from build123d import *

# Parameters (mm, degrees)
SKETCH2_R      = 3.405
EXTRUDE1_DEPTH = 550


with BuildPart() as part:
    # Sketch2 → Extrude1 (new, symmetric)
    with BuildSketch(Plane.XY):
        with BuildLine():
            Line((-16.82, 20), (-5.635, 20))
            ThreePointArc((-5.635, 20), (-4.524842354, 19.540157646), (-4.065, 18.43))
            Line((-4.065, 18.43), (-4.065, 17.51))
            ThreePointArc((-4.065, 17.51), (-4.524842354, 16.399842354), (-5.635, 15.94))
            Line((-5.635, 15.94), (-6.855, 15.94))
            Line((-6.855, 15.94), (-6.855, 16.77))
            Line((-6.855, 16.77), (-9.015, 16.77))
            ThreePointArc((-9.015, 16.77), (-9.913025612, 16.398025612), (-10.285, 15.5))
            Line((-10.285, 15.5), (-10.285, 12.987102448))
            ThreePointArc((-10.285, 12.987102448), (-10.217252784, 12.646514194), (-10.024325035, 12.357777413))
            Line((-10.024325035, 12.357777413), (-6.737790411, 9.071242789))
            ThreePointArc((-6.737790411, 9.071242789), (-5.196779505, 8.041572221), (-3.379033201, 7.68))
            Line((-3.379033201, 7.68), (3.379033201, 7.68))
            ThreePointArc((3.379033201, 7.68), (5.196779505, 8.041572221), (6.737790411, 9.071242789))
            Line((6.737790411, 9.071242789), (10.024325035, 12.357777413))
            ThreePointArc((10.024325035, 12.357777413), (10.217252784, 12.646514194), (10.285, 12.987102448))
            Line((10.285, 12.987102448), (10.285, 15.5))
            ThreePointArc((10.285, 15.5), (9.913025612, 16.398025612), (9.015, 16.77))
            Line((9.015, 16.77), (6.855, 16.77))
            Line((6.855, 16.77), (6.855, 15.94))
            Line((6.855, 15.94), (5.635, 15.94))
            ThreePointArc((5.635, 15.94), (4.524842354, 16.399842354), (4.065, 17.51))
            Line((4.065, 17.51), (4.065, 18.43))
            ThreePointArc((4.065, 18.43), (4.524842354, 19.540157646), (5.635, 20))
            Line((5.635, 20), (16.82, 20))
            ThreePointArc((16.82, 20), (19.068599564, 19.068599564), (20, 16.82))
            Line((20, 16.82), (20, 5.635))
            ThreePointArc((20, 5.635), (19.540157646, 4.524842354), (18.43, 4.065))
            Line((18.43, 4.065), (17.51, 4.065))
            ThreePointArc((17.51, 4.065), (16.399842354, 4.524842354), (15.94, 5.635))
            Line((15.94, 5.635), (15.94, 6.855))
            Line((15.94, 6.855), (16.77, 6.855))
            Line((16.77, 6.855), (16.77, 9.015))
            ThreePointArc((16.77, 9.015), (16.398025612, 9.913025612), (15.5, 10.285))
            Line((15.5, 10.285), (12.987102448, 10.285))
            ThreePointArc((12.987102448, 10.285), (12.646514194, 10.217252784), (12.357777413, 10.024325035))
            Line((12.357777413, 10.024325035), (9.071242789, 6.737790411))
            ThreePointArc((9.071242789, 6.737790411), (8.041572221, 5.196779505), (7.68, 3.379033201))
            Line((7.68, 3.379033201), (7.68, -3.379033201))
            ThreePointArc((7.68, -3.379033201), (8.041572221, -5.196779505), (9.071242789, -6.737790411))
            Line((9.071242789, -6.737790411), (12.357777413, -10.024325035))
            ThreePointArc((12.357777413, -10.024325035), (12.646514194, -10.217252784), (12.987102448, -10.285))
            Line((12.987102448, -10.285), (15.5, -10.285))
            ThreePointArc((15.5, -10.285), (16.398025612, -9.913025612), (16.77, -9.015))
            Line((16.77, -9.015), (16.77, -6.855))
            Line((16.77, -6.855), (15.94, -6.855))
            Line((15.94, -6.855), (15.94, -5.635))
            ThreePointArc((15.94, -5.635), (16.399842354, -4.524842354), (17.51, -4.065))
            Line((17.51, -4.065), (18.43, -4.065))
            ThreePointArc((18.43, -4.065), (19.540157646, -4.524842354), (20, -5.635))
            Line((20, -5.635), (20, -16.82))
            ThreePointArc((20, -16.82), (19.068599564, -19.068599564), (16.82, -20))
            Line((16.82, -20), (5.635, -20))
            ThreePointArc((5.635, -20), (4.524842354, -19.540157646), (4.065, -18.43))
            Line((4.065, -18.43), (4.065, -17.51))
            ThreePointArc((4.065, -17.51), (4.524842354, -16.399842354), (5.635, -15.94))
            Line((5.635, -15.94), (6.855, -15.94))
            Line((6.855, -15.94), (6.855, -16.77))
            Line((6.855, -16.77), (9.015, -16.77))
            ThreePointArc((9.015, -16.77), (9.913025612, -16.398025612), (10.285, -15.5))
            Line((10.285, -15.5), (10.285, -12.987102448))
            ThreePointArc((10.285, -12.987102448), (10.217252784, -12.646514194), (10.024325035, -12.357777413))
            Line((10.024325035, -12.357777413), (6.737790411, -9.071242789))
            ThreePointArc((6.737790411, -9.071242789), (5.196779505, -8.041572221), (3.379033201, -7.68))
            Line((3.379033201, -7.68), (-3.379033201, -7.68))
            ThreePointArc((-3.379033201, -7.68), (-5.196779505, -8.041572221), (-6.737790411, -9.071242789))
            Line((-6.737790411, -9.071242789), (-10.024325035, -12.357777413))
            ThreePointArc((-10.024325035, -12.357777413), (-10.217252784, -12.646514194), (-10.285, -12.987102448))
            Line((-10.285, -12.987102448), (-10.285, -15.5))
            ThreePointArc((-10.285, -15.5), (-9.913025612, -16.398025612), (-9.015, -16.77))
            Line((-9.015, -16.77), (-6.855, -16.77))
            Line((-6.855, -16.77), (-6.855, -15.94))
            Line((-6.855, -15.94), (-5.635, -15.94))
            ThreePointArc((-5.635, -15.94), (-4.524842354, -16.399842354), (-4.065, -17.51))
            Line((-4.065, -17.51), (-4.065, -18.43))
            ThreePointArc((-4.065, -18.43), (-4.524842354, -19.540157646), (-5.635, -20))
            Line((-5.635, -20), (-16.82, -20))
            ThreePointArc((-16.82, -20), (-19.068599564, -19.068599564), (-20, -16.82))
            Line((-20, -16.82), (-20, -5.635))
            ThreePointArc((-20, -5.635), (-19.540157646, -4.524842354), (-18.43, -4.065))
            Line((-18.43, -4.065), (-17.51, -4.065))
            ThreePointArc((-17.51, -4.065), (-16.399842354, -4.524842354), (-15.94, -5.635))
            Line((-15.94, -5.635), (-15.94, -6.855))
            Line((-15.94, -6.855), (-16.77, -6.855))
            Line((-16.77, -6.855), (-16.77, -9.015))
            ThreePointArc((-16.77, -9.015), (-16.398025612, -9.913025612), (-15.5, -10.285))
            Line((-15.5, -10.285), (-12.987102448, -10.285))
            ThreePointArc((-12.987102448, -10.285), (-12.646514194, -10.217252784), (-12.357777413, -10.024325035))
            Line((-12.357777413, -10.024325035), (-9.071242789, -6.737790411))
            ThreePointArc((-9.071242789, -6.737790411), (-8.041572221, -5.196779505), (-7.68, -3.379033201))
            Line((-7.68, -3.379033201), (-7.68, 3.379033201))
            ThreePointArc((-7.68, 3.379033201), (-8.041572221, 5.196779505), (-9.071242789, 6.737790411))
            Line((-9.071242789, 6.737790411), (-12.357777413, 10.024325035))
            ThreePointArc((-12.357777413, 10.024325035), (-12.646514194, 10.217252784), (-12.987102448, 10.285))
            Line((-12.987102448, 10.285), (-15.5, 10.285))
            ThreePointArc((-15.5, 10.285), (-16.398025612, 9.913025612), (-16.77, 9.015))
            Line((-16.77, 9.015), (-16.77, 6.855))
            Line((-16.77, 6.855), (-15.94, 6.855))
            Line((-15.94, 6.855), (-15.94, 5.635))
            ThreePointArc((-15.94, 5.635), (-16.399842354, 4.524842354), (-17.51, 4.065))
            Line((-17.51, 4.065), (-18.43, 4.065))
            ThreePointArc((-18.43, 4.065), (-19.540157646, 4.524842354), (-20, 5.635))
            Line((-20, 5.635), (-20, 16.82))
            ThreePointArc((-20, 16.82), (-19.068599564, 19.068599564), (-16.82, 20))
        make_face()
        Circle(SKETCH2_R, mode=Mode.SUBTRACT)
        with BuildLine():
            Line((-16.78, 18.35), (-12.575, 18.35))
            ThreePointArc((-12.575, 18.35), (-12.12245166, 18.16254834), (-11.935, 17.71))
            Line((-11.935, 17.71), (-11.935, 13.205))
            ThreePointArc((-11.935, 13.205), (-12.306974388, 12.306974388), (-13.205, 11.935))
            Line((-13.205, 11.935), (-17.71, 11.935))
            ThreePointArc((-17.71, 11.935), (-18.16254834, 12.12245166), (-18.35, 12.575))
            Line((-18.35, 12.575), (-18.35, 16.78))
            ThreePointArc((-18.35, 16.78), (-17.890157646, 17.890157646), (-16.78, 18.35))
        make_face(mode=Mode.SUBTRACT)
        with BuildLine():
            Line((-18.35, -16.78), (-18.35, -12.575))
            ThreePointArc((-18.35, -12.575), (-18.16254834, -12.12245166), (-17.71, -11.935))
            Line((-17.71, -11.935), (-13.205, -11.935))
            ThreePointArc((-13.205, -11.935), (-12.306974388, -12.306974388), (-11.935, -13.205))
            Line((-11.935, -13.205), (-11.935, -17.71))
            ThreePointArc((-11.935, -17.71), (-12.12245166, -18.16254834), (-12.575, -18.35))
            Line((-12.575, -18.35), (-16.78, -18.35))
            ThreePointArc((-16.78, -18.35), (-17.890157646, -17.890157646), (-18.35, -16.78))
        make_face(mode=Mode.SUBTRACT)
        with BuildLine():
            Line((16.78, -18.35), (12.575, -18.35))
            ThreePointArc((12.575, -18.35), (12.12245166, -18.16254834), (11.935, -17.71))
            Line((11.935, -17.71), (11.935, -13.205))
            ThreePointArc((11.935, -13.205), (12.306974388, -12.306974388), (13.205, -11.935))
            Line((13.205, -11.935), (17.71, -11.935))
            ThreePointArc((17.71, -11.935), (18.16254834, -12.12245166), (18.35, -12.575))
            Line((18.35, -12.575), (18.35, -16.78))
            ThreePointArc((18.35, -16.78), (17.890157646, -17.890157646), (16.78, -18.35))
        make_face(mode=Mode.SUBTRACT)
        with BuildLine():
            Line((18.35, 16.78), (18.35, 12.575))
            ThreePointArc((18.35, 12.575), (18.16254834, 12.12245166), (17.71, 11.935))
            Line((17.71, 11.935), (13.205, 11.935))
            ThreePointArc((13.205, 11.935), (12.306974388, 12.306974388), (11.935, 13.205))
            Line((11.935, 13.205), (11.935, 17.71))
            ThreePointArc((11.935, 17.71), (12.12245166, 18.16254834), (12.575, 18.35))
            Line((12.575, 18.35), (16.78, 18.35))
            ThreePointArc((16.78, 18.35), (17.890157646, 17.890157646), (18.35, 16.78))
        make_face(mode=Mode.SUBTRACT)
    extrude(amount=EXTRUDE1_DEPTH, both=True)


solid = part.part
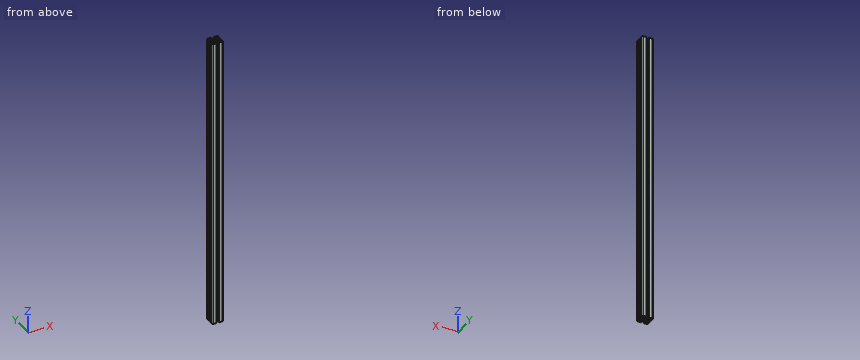
Geometry check sheet. Reference: the model listing, model coordinates, mm. Round coordinates to 2 decimals unless told otherwise and drop trailing zeros. Answer as CSV lines item,"result".
(1) Depth check by flat-ended pin: pin 1 Ø8 at (y, z) = (3.5, 239) entering from -X; pin 2 Ø0.5 at (y, z) = (18, -272.5) entering from -X; pin 3 Ø1 at (y, z) = (-18, 227.5) entering from +X. Enter the tip coordinate at first touch or a pass-through.
Output values:
pin 1,"stops at x = -20"
pin 2,"stops at x = -19.86"
pin 3,"stops at x = 19.93"
(2) Material ranges on line 1 along X through (y, z) = (6.5, -156); line 2 along Y through (x, z) = (-15, -500.5) (3 decimals); line 3 along Y through (x, z) = (0, -40.5) (3 decimals), recorded low to high.
Output values:
line 1,"x = -20 to -15.94, -8.85 to 8.85, 15.94 to 20"
line 2,"y = -20 to -18.35, -11.935 to -10.285, 10.285 to 11.935, 18.35 to 20"
line 3,"y = -7.68 to -3.405, 3.405 to 7.68"
(3) Cross-section at A-A, the plane z = -301. Give the number of separate pieces and of enclosed holes in the cut face, and give its area (3 significant figures).
Output values:
separate pieces,"1"
enclosed holes,"5"
area,"656 mm²"
